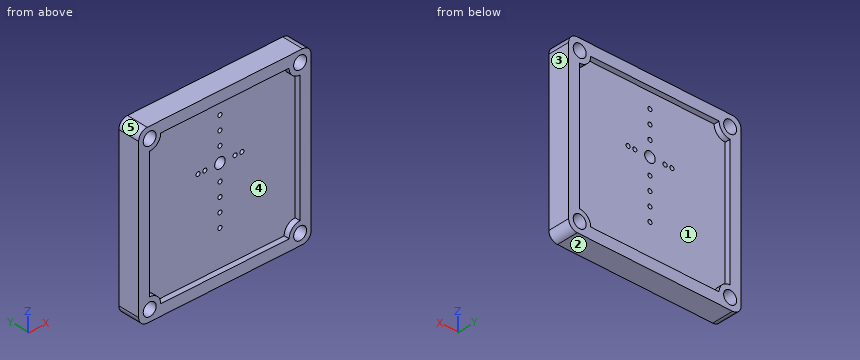
```python
from build123d import *

# Parameters (mm, degrees)
SKETCH1_W           = 50.8
SKETCH1_H           = 50.8
SKETCH1_R           = 1.905
SKETCH1_R_2         = 0.6
SKETCH1_R_3         = 1.55
BOSS_EXTRUDE1_DEPTH = 6.35
CUT_EXTRUDE1_DEPTH  = 1.5875
CUT_EXTRUDE2_START  = 4.7625
CUT_EXTRUDE2_DEPTH  = 1.5875
FILLET1_R           = 2.54


with BuildPart() as part:
    # Sketch1 → Boss-Extrude1 (new body)
    with BuildSketch(Plane(origin=(0, 0, 0), x_dir=(1, 0, 0), z_dir=(0, 1, 0))):
        with Locations((25.4, 25.4)):
            Rectangle(SKETCH1_W, SKETCH1_H)
        with Locations(Location((3.251252547, 47.548747453, 0), (0, 0, 270))):
            Circle(SKETCH1_R, mode=Mode.SUBTRACT)
        with Locations(Location((3.251252547, 3.251252547, 0), (0, 0, 270))):
            Circle(SKETCH1_R, mode=Mode.SUBTRACT)
        with Locations(Location((47.548747453, 3.251252547, 0), (0, 0, 270))):
            Circle(SKETCH1_R, mode=Mode.SUBTRACT)
        with Locations(Location((47.548747453, 47.548747453, 0), (0, 0, 270))):
            Circle(SKETCH1_R, mode=Mode.SUBTRACT)
        with Locations(Location((25.404, 11.752, 0), (0, 0, 270))):
            Circle(SKETCH1_R_2, mode=Mode.SUBTRACT)
        with Locations(Location((18.954, 20.202, 0), (0, 0, 270))):
            Circle(SKETCH1_R_2, mode=Mode.SUBTRACT)
        with Locations(Location((20.954, 20.202, 0), (0, 0, 270))):
            Circle(SKETCH1_R_2, mode=Mode.SUBTRACT)
        with Locations(Location((31.854, 20.202, 0), (0, 0, 270))):
            Circle(SKETCH1_R_2, mode=Mode.SUBTRACT)
        with Locations(Location((29.854, 20.202, 0), (0, 0, 270))):
            Circle(SKETCH1_R_2, mode=Mode.SUBTRACT)
        with Locations(Location((25.404, 37.052, 0), (0, 0, 270))):
            Circle(SKETCH1_R_2, mode=Mode.SUBTRACT)
        with Locations(Location((25.404, 33.052, 0), (0, 0, 270))):
            Circle(SKETCH1_R_2, mode=Mode.SUBTRACT)
        with Locations(Location((25.404, 29.052, 0), (0, 0, 270))):
            Circle(SKETCH1_R_2, mode=Mode.SUBTRACT)
        with Locations(Location((25.404, 25.052, 0), (0, 0, 270))):
            Circle(SKETCH1_R_2, mode=Mode.SUBTRACT)
        with Locations(Location((25.404, 7.752, 0), (0, 0, 270))):
            Circle(SKETCH1_R_2, mode=Mode.SUBTRACT)
        with Locations(Location((25.404, 15.752, 0), (0, 0, 270))):
            Circle(SKETCH1_R_2, mode=Mode.SUBTRACT)
        with Locations(Location((25.404, 20.202, 0), (0, 0, 270))):
            Circle(SKETCH1_R_3, mode=Mode.SUBTRACT)
    extrude(amount=BOSS_EXTRUDE1_DEPTH)

    # Sketch2 → Cut-Extrude1 (cut)
    with BuildSketch(Plane(origin=(0, 0, 0), x_dir=(1, 0, 0), z_dir=(0, 1, 0))):
        with BuildLine():
            ThreePointArc((6.502505094, 47.548747453), (5.55023527, 45.24976473), (3.251252547, 44.297494906))
            Line((3.251252547, 44.297494906), (3.251252547, 6.502505094))
            ThreePointArc((3.251252547, 6.502505094), (5.55023527, 5.55023527), (6.502505094, 3.251252547))
            Line((6.502505094, 3.251252547), (44.297494906, 3.251252547))
            ThreePointArc((44.297494906, 3.251252547), (45.24976473, 5.55023527), (47.548747453, 6.502505094))
            Line((47.548747453, 6.502505094), (47.548747453, 44.297494906))
            ThreePointArc((47.548747453, 44.297494906), (45.24976473, 45.24976473), (44.297494906, 47.548747453))
            Line((44.297494906, 47.548747453), (6.502505094, 47.548747453))
        make_face()
    extrude(amount=CUT_EXTRUDE1_DEPTH, mode=Mode.SUBTRACT)

    # Sketch3 → Cut-Extrude2 (cut)
    with BuildSketch(Plane(origin=(0, 0, 0), x_dir=(1, 0, 0), z_dir=(0, 1, 0)).offset(CUT_EXTRUDE2_START)):
        with BuildLine():
            ThreePointArc((6.502505094, 47.548747453), (5.55023527, 45.24976473), (3.251252547, 44.297494906))
            Line((3.251252547, 44.297494906), (3.251252547, 6.502505094))
            ThreePointArc((3.251252547, 6.502505094), (5.55023527, 5.55023527), (6.502505094, 3.251252547))
            Line((6.502505094, 3.251252547), (44.297494906, 3.251252547))
            ThreePointArc((44.297494906, 3.251252547), (45.24976473, 5.55023527), (47.548747453, 6.502505094))
            Line((47.548747453, 6.502505094), (47.548747453, 44.297494906))
            ThreePointArc((47.548747453, 44.297494906), (45.24976473, 45.24976473), (44.297494906, 47.548747453))
            Line((44.297494906, 47.548747453), (6.502505094, 47.548747453))
        make_face()
    extrude(amount=CUT_EXTRUDE2_DEPTH, mode=Mode.SUBTRACT)

    # Fillet1
    fillet1_edges = [part.edges().sort_by_distance(p)[0] for p in [
        (50.8, 3.175, -50.8),
        (50.8, 3.175, 0),
        (0, 3.175, 0),
        (0, 3.175, -50.8),
    ]]
    fillet(fillet1_edges, radius=FILLET1_R)


solid = part.part
```
The listing builds one solid part. Answer for the finished solid, in the listing's coordinates (mm). Face numbers are marked on the shaded views. A direction names the side the tool comes from. Round coordinates to 2 decimals unless told otherwise and drop trailing zeros. Loops run counter-clockwise (first coordinate to the right, second up) from the corner with the lowest first, then second, coordinate; pieces in that order, holes last. Notation, with made-up numbers: (22.5, 5) -> (65.5, 5) arc R19 ccw to (65.5, 40) -> close; hole circle Ø7 at (40, 84). An arc over 180 degrees is marked (long way). Use one line per item in the form item = value.
1. The part is cut by section C-C on z = -22.5. Determine the outline of the cut face in (x, y), and give its area (3 significant figures).
Answer key:
outline = (0, 0) -> (3.25, 0) -> (3.25, 1.59) -> (47.55, 1.59) -> (47.55, 0) -> (50.8, 0) -> (50.8, 6.35) -> (47.55, 6.35) -> (47.55, 4.76) -> (3.25, 4.76) -> (3.25, 6.35) -> (0, 6.35) -> close
area = 182 mm²
2. The part is cut by section D-D on y = 2.75. Give the number of separate pieces and of enclosed holes in the cut face, and give its area (3 significant figures).
Answer key:
separate_pieces = 1
enclosed_holes = 16
area = 2,510 mm²
3. The part is cut by section A-A on y = 5.5. Determine the outline of the cut face in (x, z) (1 decimal), and give its area (3 significant figures).
Answer key:
outline = (0, -48.3) arc R2.5 ccw to (2.5, -50.8) -> (48.3, -50.8) arc R2.5 ccw to (50.8, -48.3) -> (50.8, -2.5) arc R2.5 ccw to (48.3, 0) -> (2.5, 0) arc R2.5 ccw to (0, -2.5) -> close; hole circle Ø3.8 at (3.3, -47.5); hole circle Ø3.8 at (3.3, -3.3); hole (3.3, -44.3) arc R3.3 cw to (6.5, -47.5) -> (44.3, -47.5) arc R3.3 cw to (47.5, -44.3) -> (47.5, -6.5) arc R3.3 cw to (44.3, -3.3) -> (6.5, -3.3) arc R3.3 cw to (3.3, -6.5) -> close; hole circle Ø3.8 at (47.5, -47.5); hole circle Ø3.8 at (47.5, -3.3)
area = 600 mm²
4. Find the intervals of material crossed by probe 1 along Z at (x, y) = (26, 5); probe 2 along X at (y, z) = (5.75, -24); probe 3 along X at (y, z) = (3, -46), in increasing order. Write a range as [from, to].
Answer key:
probe_1 = [-50.8, -47.55], [-3.25, 0]
probe_2 = [0, 3.25], [47.55, 50.8]
probe_3 = [0, 2.14], [4.36, 46.44], [48.66, 50.8]
5. A tool of negligible diameter and unlimited length cuts with its end or side. For the marked faces 4 and 5, from which of +Z, -Z, +X, -X, +Y, -Y can it reach the whole face along a straight path? Write none if from no direction.
Answer key:
face_4 = -Y
face_5 = +Z, -X, +Y, -Y
6. Flat-ended cylindrical pins translate along their axes: pin 1 Ø6 at (x, z) = (9.5, -20) entering from +Y; pin 2 Ø6 at (x, z) = (3.25, -3.25) entering from -Y; pin 3 Ø22 at (x, z) = (35, -28.5) entering from -Y. Find the tip coordinate at first contact, or state that the pin passes through.
Answer key:
pin_1 = 4.76
pin_2 = 0
pin_3 = 1.59
7. For a pull along Z with two mould halves and no side action, classify the marked faces 1, 2 and 3 as released by +Z, released by -Z, zero draft, split by the parting line, or undercut.
Answer key:
face_1 = undercut
face_2 = released by -Z
face_3 = zero draft
8. The part is cut by section B-B on x = 9.5. Determine the outline of the cut face in (y, z).
Answer key:
outline = (0, -50.8) -> (6.35, -50.8) -> (6.35, -47.55) -> (4.76, -47.55) -> (4.76, -3.25) -> (6.35, -3.25) -> (6.35, 0) -> (0, 0) -> (0, -3.25) -> (1.59, -3.25) -> (1.59, -47.55) -> (0, -47.55) -> close
